Verification items for the finished model (mm, model axes). Face numbers are marked on the shaded views. A direction names the side the tool comes from. Round coordinates to 2 decimals unless told otherwise and drop trailing zeros. Loops run counter-clockwise (first coordinate to the right, second up) from the corner with the lowest first, then second, coordinate; pieces in that order, holes last. Notation, with made-up numbers: M -8,21.25 L 1,21.25 A32 ccw 1,54.25 Z; hole C 6,40 d10. An arc over 180 degrees is marked long. Answer as CSV lines item,"result".
```python
from build123d import *

# Parameters (mm, degrees)
F1_ANGLE = 180
F2_DEPTH = 33.909
F3_W     = 4.064
F3_H     = 6.35
F4_DEPTH = 29.465
F5_R     = 2.413
F6_DEPTH = 4.826
F8_DEPTH = 25.4


with BuildPart() as f1:
    # F0 (on Front) → F1 (revolve)
    with BuildSketch(Plane.XZ):
        Polygon((-14.732, 0), (0, 0), (0, 5.08), (-11.684, 5.08), (-11.684, 11.43), (-9.017, 11.43), (-9.017, 14.605), (-14.732, 14.605), align=None)
    revolve(axis=Axis((0, 0, 6.597309), (0, 0, -1)), revolution_arc=F1_ANGLE)

    # F1_face (on face) → F2 (join)
    with BuildSketch(Plane(origin=(0, 0, 5.216983), x_dir=(1, 0, 0), z_dir=(0, -1, 0))):
        Polygon((-14.732, -5.216983), (14.732, -5.216983), (14.732, 9.388017), (9.017, 9.388017), (9.017, 6.213017), (11.684, 6.213017), (11.684, -0.136983), (-11.684, -0.136983), (-11.684, 6.213017), (-9.017, 6.213017), (-9.017, 9.388017), (-14.732, 9.388017), align=None)
    extrude(amount=F2_DEPTH)

    # F3 (on face) → F4 (cut, through all)
    with BuildSketch(Plane.YZ.offset(14.732)):
        with Locations((-28.067, 8.255)):
            Rectangle(F3_W, F3_H)
    extrude(amount=-F4_DEPTH, mode=Mode.SUBTRACT)

    # F5 (on Right) → F6 (join, symmetric)
    with BuildSketch(Plane.YZ):
        with BuildLine():
            Line((-3.429, -7.62), (-3.429, 0))
            Line((-3.429, 0), (-18.669, 0))
            Line((-18.669, 0), (-18.669, -7.62))
            ThreePointArc((-18.669, -7.62), (-16.437154, -13.008154), (-11.049, -15.24))
            ThreePointArc((-11.049, -15.24), (-5.660846, -13.008154), (-3.429, -7.62))
        make_face()
        with Locations((-11.049, -7.62)):
            Circle(F5_R, mode=Mode.SUBTRACT)
    extrude(amount=F6_DEPTH, both=True)

    # F7 (on face) → F8 (cut)
    with BuildSketch(Plane.XZ.offset(18.669)):
        Polygon((1.5875, 0), (-1.5875, 0), (-1.5875, -7.62), (0, -7.62), (1.5875, -7.62), align=None)
        Polygon((0, -7.62), (-1.5875, -7.62), (-1.5875, -17.78), (1.5875, -17.78), (1.5875, -7.62), align=None)
    extrude(amount=-F8_DEPTH, mode=Mode.SUBTRACT)


solid = f1.part
```
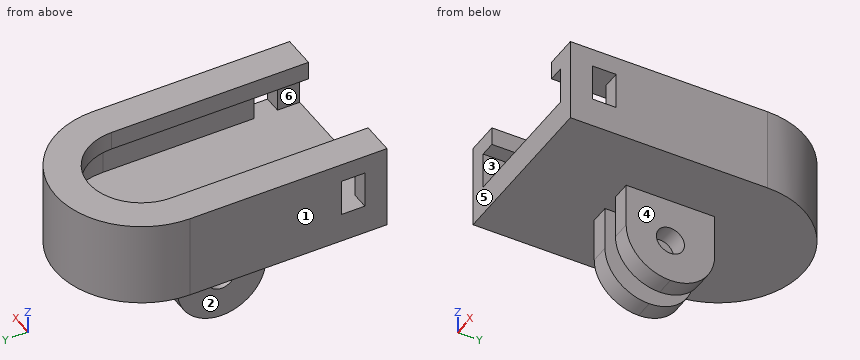
1) Material ranges on probe 1 along X at (y, z) = (-6.5, -3); probe 2 along Y at (x, z) = (-3.95, -7.62); probe 3 along X at (y, z) = (-10, 8.75), recorded low to high.
Here are the results:
probe 1,"x = -4.83 to -1.59, 1.59 to 4.83"
probe 2,"y = -18.67 to -13.46, -8.64 to -3.43"
probe 3,"x = -14.73 to -11.68, 11.68 to 14.73"
2) Set-up check for the marked faces 1, 2 and 3: record each of +Z, -Z, +X, -X, +Y, -Y from which the full face is reachable in a straight line by a thin tool's end or side.
Here are the results:
face 1,"+Z, -Z, -X, +Y, -Y"
face 2,"-Z, -X, +Y, -Y"
face 3,"-Y"
3) Section check C-C (z = -6.25). Record the cut outline in (x, y).
Here are the results:
outline,"M -4.83,-18.67 L -1.59,-18.67 L -1.59,-13.04 L -4.83,-13.04 Z; M -4.83,-9.06 L -1.59,-9.06 L -1.59,-3.43 L -4.83,-3.43 Z; M 1.59,-18.67 L 4.83,-18.67 L 4.83,-13.04 L 1.59,-13.04 Z; M 1.59,-9.06 L 4.83,-9.06 L 4.83,-3.43 L 1.59,-3.43 Z"
4) Go/stop test with flat-tipped pins: pin 1 (1.6 mm diameter, centred on x = 3.5, z = -3.5, fed in from +Y); pin 2 (4 mm diameter, centred on x = 4, y = -17, fed in from +Z); pin 3 (3 mm diameter, centred on x = 3, y = -7, fed in from -Z). Record where each tip stops, or that it passes through.
Here are the results:
pin 1,"stops at y = -3.43"
pin 2,"stops at z = 5.08"
pin 3,"stops at z = -14.8"
5) Section check D-D (z = -11.75). Record the cut outline in (x, y).
Here are the results:
outline,"M -4.83,-17.45 L -1.59,-17.45 L -1.59,-4.65 L -4.83,-4.65 Z; M 1.59,-17.45 L 4.83,-17.45 L 4.83,-4.65 L 1.59,-4.65 Z"
6) Draft check along X on the marked faces 4, 5 and 6. Enter one of: +X half, -X half, draft (parallel to the pull), parting line (faces both ways), or undercut.
Here are the results:
face 4,"+X half"
face 5,"draft"
face 6,"undercut"
7) Section check A-A (z = 7.75). Record the cut outline in (x, y) (3 decimals).
Here are the results:
outline,"M -14.732,-33.909 L -11.684,-33.909 L -11.684,-30.099 L -14.732,-30.099 Z; M -14.732,-26.035 L -11.684,-26.035 L -11.684,0 A11.684 cw 11.684,0 L 11.684,-26.035 L 14.732,-26.035 L 14.732,0 A14.732 ccw -14.732,0 Z; M 11.684,-33.909 L 14.732,-33.909 L 14.732,-30.099 L 11.684,-30.099 Z"
8) Section check B-B (x = 0). Record the cut outline in (y, z) (3 decimals), plus the area to 3 significant figures.
Here are the results:
outline,"M -33.909,0 L 14.732,0 L 14.732,14.605 L 9.017,14.605 L 9.017,11.43 L 11.684,11.43 L 11.684,5.08 L -33.909,5.08 Z"
area,"285 mm^2"
